Can you work these out from the model? Positions are in its coordinate system, mm. Face numbers are marked on the shaded views. A direction names the side the tool comes from. Give positions to 0.01 mm unless a question says otherwise; leave off trailing zeros. Loops run counter-clockwise (first coordinate to the right, second up) from the corner with the lowest first, then second, coordinate; pieces in that order, holes last.
from build123d import *

# Parameters (mm, degrees)
SKETCH3_W           = 50.8
SKETCH3_H           = 30.48
BOSS_EXTRUDE1_DEPTH = 6.35
SKETCH4_W           = 15.24
SKETCH4_H           = 30.48
BOSS_EXTRUDE2_DEPTH = 20
SKETCH5_R           = 4.135
CUT_EXTRUDE1_DEPTH  = 10.668
SKETCH6_R           = 2.35
CUT_EXTRUDE2_DEPTH  = 8
CUT_EXTRUDE3_START  = -10.668
SKETCH7_R           = 4.135
CUT_EXTRUDE3_DEPTH  = 10.668
SKETCH8_R           = 2.135
CUT_EXTRUDE4_DEPTH  = 8
SKETCH10_W          = 25.4
SKETCH10_H          = 25.4
SKETCH10_R          = 2.6
BOSS_EXTRUDE4_DEPTH = 5.08
CHAMFER1_SIZE       = 10.111093108
CHAMFER1_SIZE_2     = 27.78
FILLET2_R           = 4.92
SKETCH12_R          = 2.6
CUT_EXTRUDE6_DEPTH  = 48.353389985
SKETCH13_R          = 2.6
CUT_EXTRUDE7_DEPTH  = 48.353389985


with BuildPart() as part:
    # Sketch3 → Boss-Extrude1 (new body)
    with BuildSketch(Plane.YZ):
        with Locations((0, 15.24)):
            Rectangle(SKETCH3_W, SKETCH3_H)
    extrude(amount=BOSS_EXTRUDE1_DEPTH)

    # Sketch4 → Boss-Extrude2 (add)
    with BuildSketch(Plane(origin=(0, 0, 0), x_dir=(0, -1, 0), z_dir=(-1, 0, 0))):
        with Locations((-17.78, 15.24)):
            Rectangle(SKETCH4_W, SKETCH4_H)
        with Locations((17.78, 15.24)):
            Rectangle(SKETCH4_W, SKETCH4_H)
    extrude(amount=BOSS_EXTRUDE2_DEPTH)

    # Sketch5 → Cut-Extrude1 (cut)
    with BuildSketch(Plane(origin=(0, 25.4, 0), x_dir=(-1, 0, 0), z_dir=(0, 1, 0))):
        with Locations(Location((12.38, 15.24, 0), (0, 0, 90))):
            Circle(SKETCH5_R)
    extrude(amount=-CUT_EXTRUDE1_DEPTH, mode=Mode.SUBTRACT)

    # Sketch6 → Cut-Extrude2 (cut)
    with BuildSketch(Plane(origin=(0, 14.732, 0), x_dir=(-1, 0, 0), z_dir=(0, 1, 0))):
        with Locations(Location((12.38, 15.24, 0), (0, 0, 90))):
            Circle(SKETCH6_R)
    extrude(amount=-CUT_EXTRUDE2_DEPTH, mode=Mode.SUBTRACT)

    # Sketch7 → Cut-Extrude3 (cut)
    with BuildSketch(Plane.XZ.offset(25.4).offset(CUT_EXTRUDE3_START)):
        with Locations(Location((-12.38, 15.24, 0), (0, 0, 90))):
            Circle(SKETCH7_R)
    extrude(amount=CUT_EXTRUDE3_DEPTH, mode=Mode.SUBTRACT)

    # Sketch8 → Cut-Extrude4 (cut)
    with BuildSketch(Plane.XZ.offset(14.732)):
        with Locations(Location((-12.38, 15.24, 0), (0, 0, 270))):
            Circle(SKETCH8_R)
    extrude(amount=-CUT_EXTRUDE4_DEPTH, mode=Mode.SUBTRACT)

    # Sketch10 → Boss-Extrude4 (add)
    with BuildSketch(Plane.YZ.offset(6.35)):
        with Locations((0, 12.7)):
            Rectangle(SKETCH10_W, SKETCH10_H)
        with Locations(Location((0, 20.701, 0), (0, 0, 270))):
            Circle(SKETCH10_R, mode=Mode.SUBTRACT)
        with Locations(Location((0, 4.701, 0), (0, 0, 270))):
            Circle(SKETCH10_R, mode=Mode.SUBTRACT)
    extrude(amount=BOSS_EXTRUDE4_DEPTH)

    # Chamfer1
    # the kernel refuses this chamfer: 27.78, 10.111093108 mm, written as the material it takes off along each edge
    with BuildSketch(Plane(origin=(6.35, 25.4, 102.54672967), x_dir=(0.09904090225204921, -0.9950833631817487, 0), z_dir=(0, 0, -1)), Plane(origin=(6.35, -25.4, -72.06672967), x_dir=(0.09904090225204921, 0.9950833631817487, 0), z_dir=(0, 0, 1))) as chamfer1_piece_1:
        Polygon((CHAMFER1_SIZE * 0.995083363173, CHAMFER1_SIZE * 0.0990409022512), (-CHAMFER1_SIZE_2 * 0.099040902252, CHAMFER1_SIZE_2 * 0.995083363182), (0, 0), align=None)
    extrude(amount=174.613459341, mode=Mode.SUBTRACT)

    # Fillet2
    fillet2_edges = [part.edges().sort_by_distance(p)[0] for p in [
        (11.43, -12.7, 12.7),
        (11.43, 12.7, 12.7),
    ]]
    fillet(fillet2_edges, radius=FILLET2_R)

    # Sketch12 → Cut-Extrude6 (cut, through all)
    with BuildSketch(Plane.YZ.offset(6.35)):
        with Locations(Location((0, 20.701, 0), (0, 0, 270))):
            Circle(SKETCH12_R)
    extrude(amount=-CUT_EXTRUDE6_DEPTH, mode=Mode.SUBTRACT)

    # Sketch13 → Cut-Extrude7 (cut, through all)
    with BuildSketch(Plane.YZ.offset(6.35)):
        with Locations(Location((0, 4.701, 0), (0, 0, 270))):
            Circle(SKETCH13_R)
    extrude(amount=-CUT_EXTRUDE7_DEPTH, mode=Mode.SUBTRACT)


solid = part.part
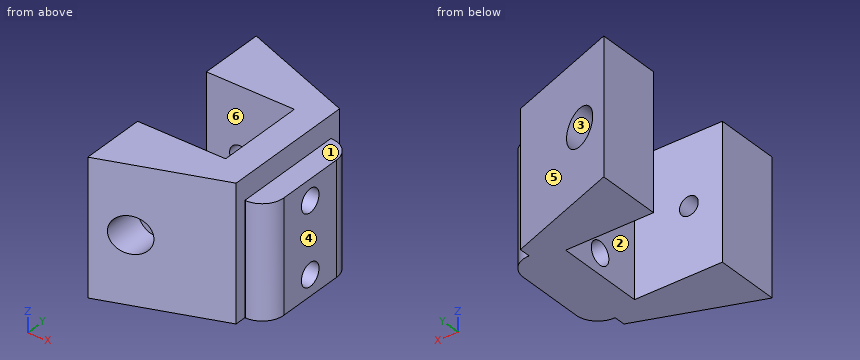
(1) Will these pins go through, and if not, where does the flat tip stop? P1, Ø9, axis at x = -11.5, z = 13.5, coming from the -Y side; P2, Ø6, axis at y = -0.5, z = 13, coming from the -X side; P3, Ø5, axis at x = -10, z = 12, coming from the -Y side.
Returned:
P1: stops at y = -23.42
P2: stops at x = 0
P3: stops at y = -22.09
(2) Suppose I cut it at B-B on x = -11. List the corners of the cut face in (y, z) for me.
Returned:
outline: (-21.6, 0) - (-10.16, 0) - (-10.16, 13.61) - (-14.73, 13.61) - (-14.73, 11.34) - (-21.6, 11.34) - close; (-21.6, 19.14) - (-14.73, 19.14) - (-14.73, 16.87) - (-10.16, 16.87) - (-10.16, 30.48) - (-21.6, 30.48) - close; (10.16, 0) - (21.6, 0) - (21.6, 11.34) - (14.73, 11.34) - (14.73, 13.34) - (10.16, 13.34) - close; (10.16, 17.14) - (14.73, 17.14) - (14.73, 19.14) - (21.6, 19.14) - (21.6, 30.48) - (10.16, 30.48) - close
(3) Please list where these lines run through material, in increasing order: probe 1 along Z at (x, y) = (-12.5, 14.5); probe 2 along X at (y, z) = (8, 8.5); probe 3 along Z at (x, y) = (-12.38, 17.75) (3 decimals).
Returned:
probe 1: z = 0 to 12.89, 17.59 to 30.48
probe 2: x = 0 to 11.43
probe 3: z = 0 to 11.105, 19.375 to 30.48
(4) Suppose I cut it at A-A on y = 0. List the corners of the cut face in (x, z) for me.
Returned:
outline: (0, 0) - (11.43, 0) - (11.43, 2.1) - (0, 2.1) - close; (0, 7.3) - (11.43, 7.3) - (11.43, 18.1) - (0, 18.1) - close; (0, 23.3) - (11.43, 23.3) - (11.43, 25.4) - (6.35, 25.4) - (6.35, 30.48) - (0, 30.48) - close
(5) Thinking about a two-plate mould opening in Y: for the marked faces 4, 5 and 6, which applies, pulls with the +Y half, pulls with the -Y half, needs draft (parallel to the pull), parting line crosses it, or undercut?
Returned:
face 4: needs draft
face 5: pulls with the +Y half
face 6: undercut
(6) Suppose I cut it at C-C on z = 15.24. Give the number of separate pieces and of enclosed holes in the cut face, plus the area to 3 significant figures.
Returned:
separate pieces: 3
enclosed holes: 0
area: 608 mm2
(7) Which directions (+Z, -Z, +X, -X, +Y, -Y) give clear straight access to the entire face, cutting with the end or side of a thin tool? Please do the marked faces 1, 2 and 3.
Returned:
face 1: +Z, +X, +Y, -Y
face 2: +Z, -Z, -X
face 3: +Y
(8) Suppose I cut it at D-D on y = -14. List the corners of the cut face in (x, z) for me (3 decimals).
Returned:
outline: (-20, 0) - (6.35, 0) - (6.35, 30.48) - (-20, 30.48) - close; hole circle Ø4.27 at (-12.38, 15.24)
